```python
from build123d import *

# Parameters (mm, degrees)
F0_W     = 10
F0_H     = 115
F0_W_2   = 25.3
F0_H_2   = 18
F1_DEPTH = 2
F3_W     = 2.7
F3_H     = 18
F3_W_2   = 18
F3_H_2   = 2.7
F4_DEPTH = 7
F5_R     = 4.99999


# Not quite as in the source:
# - a fillet or chamfer is up to 0.001 mm smaller than in the source, because OpenCascade refuses the exact size


with BuildPart() as f1:
    # F0 (on Top) → F1 (new body)
    with BuildSketch(Plane.XY):
        Polygon((9, 135.3739356415), (-9, 135.3739356415), (-9, 83.5739356415), (-9, 65.5739356415), (-9, -4.2260643585), (9, -4.2260643585), (9, 65.5739356415), (9, 83.5739356415), align=None)
        with Locations((0, 63.2739356415)):
            Rectangle(F0_W, F0_H, mode=Mode.SUBTRACT)
        with Locations((-21.65, 74.5739356415)):
            Rectangle(F0_W_2, F0_H_2)
        with Locations((21.65, 74.5739356415)):
            Rectangle(F0_W_2, F0_H_2)
    extrude(amount=F1_DEPTH)

    # F3 (on face) → F4 (join)
    with BuildSketch(Plane.XY.offset(2)):
        with Locations((-32.95, 74.5739356415)):
            Rectangle(F3_W, F3_H)
        with Locations((32.95, 74.5739356415)):
            Rectangle(F3_W, F3_H)
        with Locations((0, 134.0239356415)):
            Rectangle(F3_W_2, F3_H_2)
        with Locations((0, -2.8760643585)):
            Rectangle(F3_W_2, F3_H_2)
    extrude(amount=F4_DEPTH)

    # F5 (radius 5 in the source; OpenCascade refuses exactly that, so slightly less here)
    f5_edges = [f1.edges().sort_by_distance(p)[0] for p in [
        (-9, 65.573936, 1),
        (9, 65.573936, 1),
        (9, 83.573936, 1),
        (-9, 83.573936, 1),
        (-5, 120.773936, 1),
        (5, 120.773936, 1),
    ]]
    fillet(f5_edges, radius=F5_R)


solid = f1.part
```
Here's how the part is built. I have some questions about the finished solid (model axes, mm). A direction names the side the tool comes from. Coordinates: 2 decimals unless noted, no trailing zeros. Write each loop counter-clockwise with the first axis right and the second up, starting at its lowest first coordinate (ties: lowest second). Pieces come first, ordered by that corner, then holes. Notation, with made-up numbers: (34, 84) -> (53, 84) arc R22 cw to (53, 119) -> close; hole circle Ø11 at (56.5, 46.5). An arc over 180 degrees is marked (long way). Use a Markdown table: item, result. Add a question column.
(1) Please list where these lines run through material, in increasing order: line 1 (X direction, y = 54, z = 1.25); line 2 (Y direction, x = -0.5, z = 1.25); line 3 (Y direction, x = 7, z = 7.5).
(2) For faces 1 (the flat face through (0, 132.674, 5)), 2 (the flat face through (26.4, 83.574, 1.8)), 3 (the flat face through (26.4, 65.574, 1.8)), which set-ups out of +Z, -Z, +X, -X, +Y, -Y let a thin tool reach every point of the face, with its end or its side?
(3) If we section it at C-C, the plane y = 69.5: Write out the boundary of the cut face in (x, z).
(4) I'm going to push flat-ended pins straight in: P1, Ø4.5, axis at x = 26, z = 3.5, coming from the +Y side; P2, Ø2.5, axis at x = 25.5, z = 2.5, coming from the -Y side; P3, Ø5, axis at y = 48.5, z = 1.5, coming from the +X side. Where does each tip first touch, or does it pass through?
(5) If we section it at D-D, the plane x = -28: Write out the boundary of the cut face in (y, z).
(6) If we section it at A-A, the plane y = 52.5: Write out the boundary of the cut face in (x, z).
(7) If we section it at B-B, the plane z = 5.5: Write out the boundary of the cut face in (x, y), and give its area (3 significant figures).
(8) We'd pull the mould along Y, two halves only. Please class faces 4 (the cylindrical face through (10.504, 85, 1.014)), 5 (the flat face through (0, -1.526, 5)), 6 (the flat face through (-31.6, 74, 5)), 7 (the cylindrical face through (-3.496, 119.348, 1.014)): +Y half, -Y half, draft (parallel to the pull), parting line (faces both ways), or undercut.
Outcome:
| question | item | result |
|---|---|---|
| 1 | line 1 | x = -9 to -5, 5 to 9 |
| 1 | line 2 | y = -4.23 to 5.77, 120.75 to 135.37 |
| 1 | line 3 | y = -4.23 to -1.53, 132.67 to 135.37 |
| 2 | face 1 | +Z, +X, -X |
| 2 | face 2 | +Z, -Z, +X, +Y |
| 2 | face 3 | +Z, -Z, +X, -Y |
| 3 | outline | (-34.3, 0) -> (-5, 0) -> (-5, 2) -> (-31.6, 2) -> (-31.6, 9) -> (-34.3, 9) -> close; (5, 0) -> (34.3, 0) -> (34.3, 9) -> (31.6, 9) -> (31.6, 2) -> (5, 2) -> close |
| 4 | P1 | stops at y = 83.57 |
| 4 | P2 | stops at y = 65.57 |
| 4 | P3 | stops at x = 9 |
| 5 | outline | (65.57, 0) -> (83.57, 0) -> (83.57, 2) -> (65.57, 2) -> close |
| 6 | outline | (-9, 0) -> (-5, 0) -> (-5, 2) -> (-9, 2) -> close; (5, 0) -> (9, 0) -> (9, 2) -> (5, 2) -> close |
| 7 | outline | (-34.3, 65.57) -> (-31.6, 65.57) -> (-31.6, 83.57) -> (-34.3, 83.57) -> close; (-9, -4.23) -> (9, -4.23) -> (9, -1.53) -> (-9, -1.53) -> close; (-9, 132.67) -> (9, 132.67) -> (9, 135.37) -> (-9, 135.37) -> close; (31.6, 65.57) -> (34.3, 65.57) -> (34.3, 83.57) -> (31.6, 83.57) -> close |
| 7 | area | 194 mm^2 |
| 8 | face 4 | +Y half |
| 8 | face 5 | undercut |
| 8 | face 6 | draft |
| 8 | face 7 | undercut |
